from build123d import *

# Parameters (mm, degrees)
F0_R     = 2.38125
F1_DEPTH = 3.175
F2_DEPTH = 4.7625
F3_T     = -1.5875
F4_R     = 3.175
F4_R_2   = 2.38125
F5_DEPTH = 1.5875


with BuildPart() as f1:
    # F0 (on Top) → F1 (new body)
    with BuildSketch(Plane.XY):
        Polygon((11.90625, 31.75), (3.96875, 31.75), (-11.90625, -15.875), (-11.90625, -31.75), (11.90625, -31.75), align=None)
        with Locations((-7.9375, -27.78125)):
            Circle(F0_R, mode=Mode.SUBTRACT)
        with Locations((-7.9375, -19.84375)):
            Circle(F0_R, mode=Mode.SUBTRACT)
        with Locations((0, -27.78125)):
            Circle(F0_R, mode=Mode.SUBTRACT)
        with Locations((0, -19.84375)):
            Circle(F0_R, mode=Mode.SUBTRACT)
        with Locations((7.9375, -27.78125)):
            Circle(F0_R, mode=Mode.SUBTRACT)
        with Locations((7.9375, -19.84375)):
            Circle(F0_R, mode=Mode.SUBTRACT)
        with Locations((0, -11.90625)):
            Circle(F0_R, mode=Mode.SUBTRACT)
        with Locations((0, -3.96875)):
            Circle(F0_R, mode=Mode.SUBTRACT)
        with Locations((7.9375, -11.90625)):
            Circle(F0_R, mode=Mode.SUBTRACT)
        with Locations((7.9375, -3.96875)):
            Circle(F0_R, mode=Mode.SUBTRACT)
        with Locations((0, 3.96875)):
            Circle(F0_R, mode=Mode.SUBTRACT)
        with Locations((7.9375, 3.96875)):
            Circle(F0_R, mode=Mode.SUBTRACT)
        with Locations((7.9375, 11.90625)):
            Circle(F0_R, mode=Mode.SUBTRACT)
        with Locations((7.9375, 19.84375)):
            Circle(F0_R, mode=Mode.SUBTRACT)
        with Locations((7.9375, 27.78125)):
            Circle(F0_R, mode=Mode.SUBTRACT)
    extrude(amount=F1_DEPTH)

    # F0 (on Top) → F2 (join)
    with BuildSketch(Plane.XY):
        with Locations((7.9375, 27.78125)):
            Circle(F0_R)
        with Locations((7.9375, 19.84375)):
            Circle(F0_R)
        with Locations((7.9375, 11.90625)):
            Circle(F0_R)
        with Locations((0, 3.96875)):
            Circle(F0_R)
        with Locations((7.9375, 3.96875)):
            Circle(F0_R)
        with Locations((7.9375, -3.96875)):
            Circle(F0_R)
        with Locations((0, -3.96875)):
            Circle(F0_R)
        with Locations((0, -11.90625)):
            Circle(F0_R)
        with Locations((7.9375, -11.90625)):
            Circle(F0_R)
        with Locations((7.9375, -19.84375)):
            Circle(F0_R)
        with Locations((0, -19.84375)):
            Circle(F0_R)
        with Locations((-7.9375, -19.84375)):
            Circle(F0_R)
        with Locations((-7.9375, -27.78125)):
            Circle(F0_R)
        with Locations((0, -27.78125)):
            Circle(F0_R)
        with Locations((7.9375, -27.78125)):
            Circle(F0_R)
    extrude(amount=F2_DEPTH)

    # F3
    f3_openings = [f1.faces().sort_by_distance(p)[0] for p in [
        (2.204861, -5.291667, 0),
    ]]
    offset(amount=F3_T, openings=f3_openings, kind=Kind.INTERSECTION)

    # F4 (on face) → F5 (join)
    with BuildSketch(Plane(origin=(0, 0, 1.5875), x_dir=(1, 0, 0), z_dir=(0, 0, -1))):
        with BuildLine():
            ThreePointArc((-0.79375, 23.8125), (-2.7537301022, 26.7458175157), (-6.2138140303, 26.0575640303))
            Line((-6.2138140303, 26.0575640303), (-5.6525480227, 25.4962980227))
            ThreePointArc((-5.6525480227, 25.4962980227), (-3.0574850767, 26.0124881368), (-1.5875, 23.8125))
            ThreePointArc((-1.5875, 23.8125), (-1.7687618632, 22.9012350767), (-2.2849519773, 22.1287019773))
            Line((-2.2849519773, 22.1287019773), (-1.7236859697, 21.5674359697))
            ThreePointArc((-1.7236859697, 21.5674359697), (-1.0354324843, 22.5974801022), (-0.79375, 23.8125))
        make_face()
        with BuildLine():
            Line((-5.6525480227, 25.4962980227), (-6.2138140303, 26.0575640303))
            ThreePointArc((-6.2138140303, 26.0575640303), (-6.2138140303, 21.5674359697), (-1.7236859697, 21.5674359697))
            Line((-1.7236859697, 21.5674359697), (-2.2849519773, 22.1287019773))
            ThreePointArc((-2.2849519773, 22.1287019773), (-5.6525480227, 22.1287019773), (-5.6525480227, 25.4962980227))
        make_face()
        with Locations((-3.96875, 15.875)):
            Circle(F4_R)
        with Locations((-3.96875, 15.875)):
            Circle(F4_R_2, mode=Mode.SUBTRACT)
        with Locations((-3.96875, 7.9375)):
            Circle(F4_R)
        with Locations((-3.96875, 7.9375)):
            Circle(F4_R_2, mode=Mode.SUBTRACT)
        with BuildLine():
            ThreePointArc((-3.8832617755, -3.1738488879), (-1.6936620772, -2.2146331397), (-0.79375, 0))
            ThreePointArc((-0.79375, 0), (-2.5107405764, 2.8204314423), (-5.8046687532, 2.590372045))
            Line((-5.8046687532, 2.590372045), (-5.5381726179, 1.7908836392))
            ThreePointArc((-5.5381726179, 1.7908836392), (-2.9856009895, 2.1688175547), (-1.5875, 0))
            ThreePointArc((-1.5875, 0), (-2.350212624, -1.7466219754), (-4.1497579108, -2.3743604821))
            Line((-4.1497579108, -2.3743604821), (-3.8832617755, -3.1738488879))
        make_face()
        with BuildLine():
            ThreePointArc((7.14375, -23.8125), (5.4267594236, -20.9920685577), (2.1328312468, -21.222127955))
            Line((2.1328312468, -21.222127955), (2.3993273821, -22.0216163608))
            ThreePointArc((2.3993273821, -22.0216163608), (4.9518990105, -21.6436824453), (6.35, -23.8125))
            ThreePointArc((6.35, -23.8125), (5.587287376, -25.5591219754), (3.7877420892, -26.1868604821))
            Line((3.7877420892, -26.1868604821), (4.0542382245, -26.9863488879))
            ThreePointArc((4.0542382245, -26.9863488879), (6.2438379228, -26.0271331397), (7.14375, -23.8125))
        make_face()
        with Locations((3.96875, 23.8125)):
            Circle(F4_R)
        with Locations((3.96875, 23.8125)):
            Circle(F4_R_2, mode=Mode.SUBTRACT)
        with Locations((3.96875, 15.875)):
            Circle(F4_R)
        with Locations((3.96875, 15.875)):
            Circle(F4_R_2, mode=Mode.SUBTRACT)
        with Locations((3.96875, 7.9375)):
            Circle(F4_R)
        with Locations((3.96875, 7.9375)):
            Circle(F4_R_2, mode=Mode.SUBTRACT)
        with Locations((3.96875, 0)):
            Circle(F4_R)
        with Locations((3.96875, 0)):
            Circle(F4_R_2, mode=Mode.SUBTRACT)
        with Locations((3.96875, -7.9375)):
            Circle(F4_R)
        with Locations((3.96875, -7.9375)):
            Circle(F4_R_2, mode=Mode.SUBTRACT)
        with Locations((3.96875, -15.875)):
            Circle(F4_R)
        with Locations((3.96875, -15.875)):
            Circle(F4_R_2, mode=Mode.SUBTRACT)
    extrude(amount=F5_DEPTH)


solid = f1.part
Here's how the part is built. I have some questions about the finished solid (model axes, mm). A direction names the side the tool comes from. Give positions to 0.01 mm unless a question says otherwise; leave off trailing zeros. Use a Markdown table: item, result. Add a question column.
Item 1: Imagine slicing it at A-A on z = 4.05. Give the number of separate pieces and of enclosed holes in the cut face, plus the area to 3 significant figures.
Item 2: If we mould it in two halves opening along X, with no side actions, what happens to faces 4 (the face through (0, 4, 3.175)), 5 (the face through (7.42, -14.23, 3.96)), 6 (the face through (8, 20, 4.762))? For each: pulls with the +X half, pulls with the -X half, needs draft (parallel to the pull), parting line crosses it, or undercut.
Item 3: For faces 1 (the face through (0, -12, 4.762)), 2 (the face through (-0.31, 6.33, 3.96)), 3 (the face through (4, 16, 1.588)), which set-ups out of +Z, -Z, +X, -X, +Y, -Y let a thin tool reach every point of the face, with its end or its side?
Item 4: I need wall thicknesses on line 1 (X direction, y = 21, z = 0.65); line 2 (Y direction, x = -1, z = 3.9); line 3 (X direction, y = 4, z = 4.4). Which ranges of each line are inside material? Lowest first, please.
Item 5: Will these pins go through, and if not, where does the flat tip stop? pin 1 (1.4 mm diameter, centred on x = 3.5, y = 15.5, fed in from -Z); pin 2 (5.5 mm diameter, centred on x = -3.97, y = -7.94, fed in from +Z) (3 decimals); pin 3 (10 mm diameter, centred on x = -4, y = -21, fed in from +Z); pin 4 (2 mm diameter, centred on y = 0.5, z = 3.5, fed in from -X).
Data:
| question | item | result |
|---|---|---|
| 1 | separate pieces | 15 |
| 1 | enclosed holes | 0 |
| 1 | area | 267 mm² |
| 2 | face 4 | undercut |
| 2 | face 5 | undercut |
| 2 | face 6 | needs draft |
| 3 | face 1 | +Z, +X, -X, +Y, -Y |
| 3 | face 2 | +Z |
| 3 | face 3 | -Z |
| 4 | line 1 | x = 0.39 to 2.06, 2.5 to 5.44, 10.32 to 11.91 |
| 4 | line 2 | y = -29.94 to -25.62, -22 to -17.68, -14.07 to -9.75, -6.13 to -1.81, 1.81 to 6.13 |
| 4 | line 3 | x = -2.38 to 2.38, 5.56 to 10.32 |
| 5 | pin 1 | stops at z = 1.59 |
| 5 | pin 2 | stops at z = 3.175 |
| 5 | pin 3 | stops at z = 4.76 |
| 5 | pin 4 | stops at x = -6.76 |
